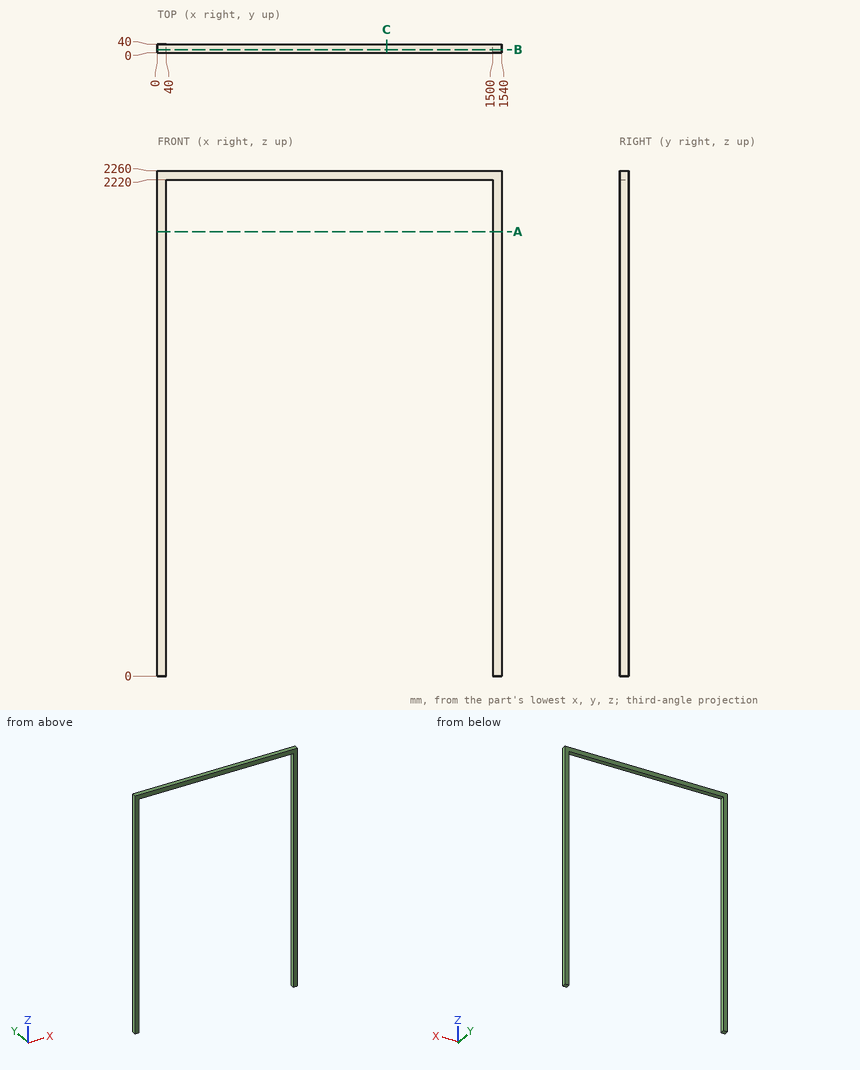
Input: dimensioned drawing with shaded views. Units: mm. Origin: part minimum x, y, z. Coordinates: 2 decimals unless noted, no trailing zeros. Order: outer loops, then holes, each group sorted by start corner. A loop starts at its lowest first (then second) coordinate and runs counter-clockwise, first axis right, second up.
1. Cut plane B-B, the plane y = 15. Return loops of the section in (x, z).
Checked values:
outline: (0, 0) - (40, 0) - (40, 2220) - (1500, 2220) - (1500, 0) - (1540, 0) - (1540, 2260) - (0, 2260) - close
2. Ray query, line 1 along X through (y, z) = (22, 1461); line 2 along Z through (x, y) = (984, 25.5). Return the intervals inside material, ascending.
Checked values:
line 1: x = 0 to 40, 1500 to 1540
line 2: z = 2220 to 2260
3. Cut plane C-C, the plane x = 1025. Return loops of the section in (y, z).
Checked values:
outline: (0, 2220) - (40, 2220) - (40, 2260) - (0, 2260) - close
4. Contact query for a flat-ended pin moving along its axis: P1, Ø6, axis at x = 204, y = 28.5, coming from the -Z side. Output: stop coordinate, or through.
Checked values:
P1: stops at z = 2220
5. Cut plane A-A, the plane z = 1988. Return loops of the section in (x, y).
Checked values:
outline: (0, 0) - (40, 0) - (40, 40) - (0, 40) - close; (1500, 0) - (1540, 0) - (1540, 40) - (1500, 40) - close
